Geometry: final body of the model. Coordinates: model frame, mm. Face numbers are marked on the shaded views. Give positions to 0.01 mm unless a question says otherwise; leave off trailing zeros. Loops run counter-clockwise (first coordinate to the right, second up) from the corner with the lowest first, then second, coordinate; pieces in that order, holes last.
from build123d import *

# Parameters (mm, degrees)
CYLINDER014_R          = 0.8
CYLINDER014_DEPTH      = 12
CYLINDER025_R          = 0.8
CYLINDER025_DEPTH      = 12
CYLINDER015_R          = 0.8
CYLINDER015_DEPTH      = 12
CYLINDER012_R          = 5
CYLINDER012_DEPTH      = 6.5
FILLET022_R            = 1
BOX017_W               = 25
BOX017_H               = 30
BOX017_DEPTH           = 8
FILLET018_R            = 9
FILLET019_R            = 5
CHAMFER001_SIZE        = 10
FILLET020_R            = 10
FILLET021_R            = 1.5
CUT010_PLACEMENT_ANGLE = 10


with BuildPart() as obj1:
    # Cylinder014 → Cylinder014 (new body)
    with BuildSketch(Plane(origin=(3, 17, 0), x_dir=(1, 0, 0), z_dir=(0, 0, 1))):
        Circle(CYLINDER014_R)
    extrude(amount=CYLINDER014_DEPTH)


with BuildPart() as obj2:
    # Cylinder025 → Cylinder025 (new body)
    with BuildSketch(Plane(origin=(11, 8, 0), x_dir=(1, 0, 0), z_dir=(0, 0, 1))):
        Circle(CYLINDER025_R)
    extrude(amount=CYLINDER025_DEPTH)


with BuildPart() as obj3:
    # Cylinder015 → Cylinder015 (new body)
    with BuildSketch(Plane(origin=(12, -4, 0), x_dir=(1, 0, 0), z_dir=(0, 0, 1))):
        Circle(CYLINDER015_R)
    extrude(amount=CYLINDER015_DEPTH)


with BuildPart() as fusion010:
    # Cylinder012 → Cylinder012 (new body)
    with BuildSketch(Plane.XY):
        Circle(CYLINDER012_R)
    extrude(amount=CYLINDER012_DEPTH)

    # Fillet022
    fillet022_edges = [fusion010.edges().sort_by_distance(p)[0] for p in [
        (-5, 0, 6.5),
    ]]
    fillet(fillet022_edges, radius=FILLET022_R)

    # Fusion010: union obj1, obj2, obj3
    add(obj1.part)
    add(obj2.part)
    add(obj3.part)


with BuildPart() as cut010:
    # Box017 → Box017 (new body)
    with BuildSketch(Plane(origin=(-9, -9, 4.5), x_dir=(1, 0, 0), z_dir=(0, 0, 1))):
        with Locations((12.5, 15)):
            Rectangle(BOX017_W, BOX017_H)
    extrude(amount=BOX017_DEPTH)

    # Fillet018
    fillet018_edges = [cut010.edges().sort_by_distance(p)[0] for p in [
        (-9, -9, 8.5),
    ]]
    fillet(fillet018_edges, radius=FILLET018_R)

    # Fillet019
    fillet019_edges = [cut010.edges().sort_by_distance(p)[0] for p in [
        (-9, 21, 8.5),
        (16, -9, 8.5),
    ]]
    fillet(fillet019_edges, radius=FILLET019_R)

    # Chamfer001
    chamfer001_edges = [cut010.edges().sort_by_distance(p)[0] for p in [
        (16, 21, 8.5),
    ]]
    chamfer(chamfer001_edges, length=CHAMFER001_SIZE)

    # Fillet020
    fillet020_edges = [cut010.edges().sort_by_distance(p)[0] for p in [
        (6, 21, 8.5),
        (16, 11, 8.5),
    ]]
    fillet(fillet020_edges, radius=FILLET020_R)

    # Fillet021
    fillet021_edges = [cut010.edges().sort_by_distance(p)[0] for p in [
        (11, 16, 12.5),
    ]]
    fillet(fillet021_edges, radius=FILLET021_R)

    # Cut010: cut Fusion010
    add(fusion010.part, mode=Mode.SUBTRACT)


with BuildPart() as cut010_1:
    # Cut010 placement: moved
    add(cut010.part.moved(Location((0, -2, 0))).rotate(Axis((0, -2, 0), (0, 0, 1)), CUT010_PLACEMENT_ANGLE))


solid = cut010_1.part
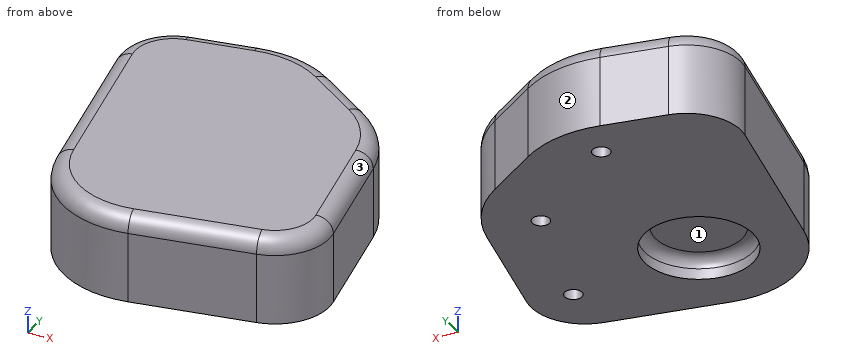
Item 1: Section query A-A on z = 7. Return loops of the section in (x, y), plus the area to 3 significant figures.
Values follow:
outline: (-11.64, 12.19) - (-8.86, -3.56) arc R9 ccw to (1.56, -10.86) - (12.4, -8.95) arc R5 ccw to (16.45, -3.16) - (14.57, 7.53) arc R10 ccw to (10.45, 13.99) - (5.66, 17.35) arc R10 ccw to (-1.82, 19) - (-7.59, 17.99) arc R5 ccw to start; hole circle Ø1.6 at (0, 15.26); hole circle Ø1.6 at (9.44, 7.79); hole circle Ø1.6 at (12.51, -3.86)
area: 662 mm2
Item 2: Ray query, probe 1 along Y at (x, z) = (0, 7); probe 2 along X at (y, z) = (1, 5.25); probe 3 along X at (y, z) = (-4, 7). Return the intervals inside material, ascending.
Values follow:
probe 1: y = -11 to 14.46, 16.06 to 19.16
probe 2: x = -9.67 to -4, 4 to 15.72
probe 3: x = -8.77 to 11.73, 13.3 to 16.53
Item 3: Pin query (flat end, axial travel): pin 1 (3 mm diameter, centred on y = 5.5, z = 7.5, fed in from -X); pin 2 (1.3 mm diameter, centred on x = 9.44, y = 7.79, fed in from -Z). Return the tip coordinate at first contact, or that it passes through.
Values follow:
pin 1: stops at x = -10.73
pin 2: stops at z = 12
Item 4: Draft query along X for the marked faces 1, 2 and 3. Return one class per face: +X half, -X half, draft (parallel to the pull), parting line (faces both ways), or undercut.
Values follow:
face 1: undercut
face 2: parting line
face 3: +X half
